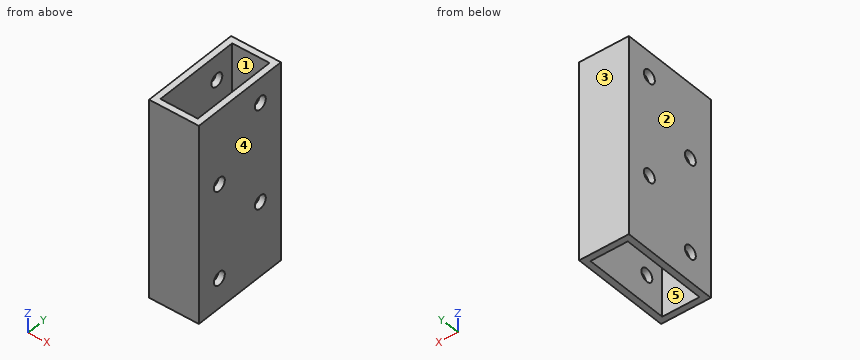
Autodesk Inventor part; units mm, degrees
ref_plane "YZ Plane" through (0, 0, 0) normal (1, 0, 0) x (0, 1, 0)
ref_plane "XZ Plane" through (0, 0, 0) normal (0, 1, 0) x (-1, 0, 0)
ref_plane "XY Plane" through (0, 0, 0) normal (0, 0, 1) x (1, 0, 0)
sketch "Sketch1" plane through (0, 0, 0) normal (0, 0, 1) x (1, 0, 0)
  line L0 (0, 0) -> (25.4, 0)
  line L1 (25.4, 0) -> (25.4, -50.8)
  line L2 (25.4, -50.8) -> (0, -50.8)
  line L3 (0, -50.8) -> (0, 0)
  line L4 (3.175, -3.175) -> (22.225, -3.175)
  line L5 (22.225, -3.175) -> (22.225, -47.625)
  line L6 (22.225, -47.625) -> (3.175, -47.625)
  line L7 (3.175, -47.625) -> (3.175, -3.175)
  dimension "d0" = 25.4
  dimension "d1" = 50.8
  dimension "d2" = 3.175
  dimension "d3" = 3.175
  dimension "d4" = 3.175
  dimension "d5" = 3.175
extrude "Extrusion1" add sketch "Sketch1" along normal blind 101.6
sketch "Sketch2" plane through (25.4, -50.8, 0) normal (1, 0, 0) x (0, 0, -1)
  circle A0 centre (-63.5, 12.7) radius 3.3734
  line L0 (0, 50.8) -> (0, 0)
  line L1 (0, 50.8) -> (-101.6, 50.8)
  circle A1 centre (-88.9, 38.1) radius 3.3734
  circle A2 centre (-38.1, 38.1) radius 3.3734
  circle A3 centre (-15.24, 12.7) radius 3.3734
  line L2 (0, 0) -> (-101.6, 0)
  dimension "d8" = 6.7469
  dimension "d12" = 63.5
  dimension "d13" = 88.9
  dimension "d14" = 12.7
  dimension "d17" = 38.1
  dimension "d27" = 15.24
  dimension "d28" = 12.7
  dimension "d29" = 38.1
  dimension "d30" = 12.7
extrude "Extrusion3" cut sketch "Sketch2" against normal blind 25.4
properties part number "flywheelsupport" material "Aluminum 6061"
Build history of the part. All positions in model axes, mm. Face numbers are marked on the shaded views. A direction names the side the tool comes from. Round coordinates to 2 decimals unless told otherwise and drop trailing zeros. Write each loop counter-clockwise with the first axis right and the second up, starting at its lowest first coordinate (ties: lowest second). Pieces come first, ordered by that corner, then holes. Notation, with made-up numbers: (41.25, 36) - (49.25, 36) arc R12 ccw to (49.25, 44) - close; hole circle Ø5 at (-4.5, -34.5). An arc over 180 degrees is marked (long way). Write each question's results on one line, items separated by ' | '. Start each with the question number.
Item 1: Saw through at D-D (y = -12.7). Write the cut outline in (x, z) (3 decimals), and give its area (3 significant figures).
Item 2: Mould opens along X. For the marked faces 1, 2 and 3 say: pulls with the +X half, pulls with the -X half, needs draft (parallel to the pull), parting line crosses it, or undercut.
Item 3: Saw through at C-C (z = 46). Write the cut outline in (x, y) (3 decimals).
Item 4: Which spindle directions (+Z, -Z, +X, -X, +Y, -Y) get a long thin tool onto all of the face, cutting with end or side? Do the marked faces 4 and 5. Say none if no direction does.
Item 5: Saw through at A-A (y = -7.5). Write the cut outline in (x, z) (3 decimals).
Item 6: Saw through at B-B (x = 11). Write the cut outline in (y, z) (3 decimals), and give its area (3 significant figures).
Item 7: Wall check: L1, parallel to Z at x = 1.5, y = -12.5; L2, parallel to X at y = -27.5, z = 16 (3 decimals); L3, parallel to Y at x = 15.75, z = 95.5 (3 decimals). Give the ranges that are in metal, low to high. Write a range as [from, to].
Results are:
1) outline: (0, 0) - (3.175, 0) - (3.175, 34.727) - (0, 34.727) - close; (0, 41.473) - (3.175, 41.473) - (3.175, 85.527) - (0, 85.527) - close; (0, 92.273) - (3.175, 92.273) - (3.175, 101.6) - (0, 101.6) - close; (22.225, 0) - (25.4, 0) - (25.4, 34.727) - (22.225, 34.727) - close; (22.225, 41.473) - (25.4, 41.473) - (25.4, 85.527) - (22.225, 85.527) - close; (22.225, 92.273) - (25.4, 92.273) - (25.4, 101.6) - (22.225, 101.6) - close | area: 559 mm²
2) face 1: undercut | face 2: pulls with the -X half | face 3: needs draft
3) outline: (0, -50.8) - (25.4, -50.8) - (25.4, 0) - (0, 0) - close; hole (3.175, -47.625) - (22.225, -47.625) - (22.225, -3.175) - (3.175, -3.175) - close
4) face 4: +Z, -Z, +X, +Y, -Y | face 5: +Z, -Z
5) outline: (0, 0) - (3.175, 0) - (3.175, 101.6) - (0, 101.6) - close; (22.225, 0) - (25.4, 0) - (25.4, 101.6) - (22.225, 101.6) - close
6) outline: (-50.8, 0) - (-47.625, 0) - (-47.625, 101.6) - (-50.8, 101.6) - close; (-3.175, 0) - (0, 0) - (0, 101.6) - (-3.175, 101.6) - close | area: 645 mm²
7) L1: z = [0, 34.73], [41.47, 85.53], [92.27, 101.6] | L2: x = [0, 3.175], [22.225, 25.4] | L3: y = [-50.8, -47.625], [-3.175, 0]
